Autodesk Inventor part; units mm, degrees
ref_plane "YZ Plane" through (0, 0, 0) normal (1, 0, 0) x (0, 1, 0)
ref_plane "XZ Plane" through (0, 0, 0) normal (0, 1, 0) x (-1, 0, 0)
ref_plane "XY Plane" through (0, 0, 0) normal (0, 0, 1) x (1, 0, 0)
sketch "Sketch1" plane through (0, 0, 0) normal (0, 0, 1) x (1, 0, 0)
  line L0 (0, 0) -> (25.6, 0)
  line L1 (25.6, 0) -> (25.6, -22)
  line L2 (25.6, -22) -> (0, -22)
  line L3 (0, -22) -> (0, 0)
  circle A0 centre (2.45, -19.55) radius 1.5
  line L4 (12.8, -22) -> (12.8, -20.4874)
  circle A1 centre (23.15, -19.55) radius 1.5
  circle A2 centre (5, -3.2) radius 1.5
  dimension "d0" = 25.6
  dimension "d1" = 22
  dimension "d2" = 3
  dimension "d3" = 2.45
  dimension "d4" = 2.45
  dimension "d5" = 3.2
  dimension "d6" = 3
extrude "Extrusion1" add sketch "Sketch1" along normal blind 2
properties part number "Plate_SEN_Current_sensor"
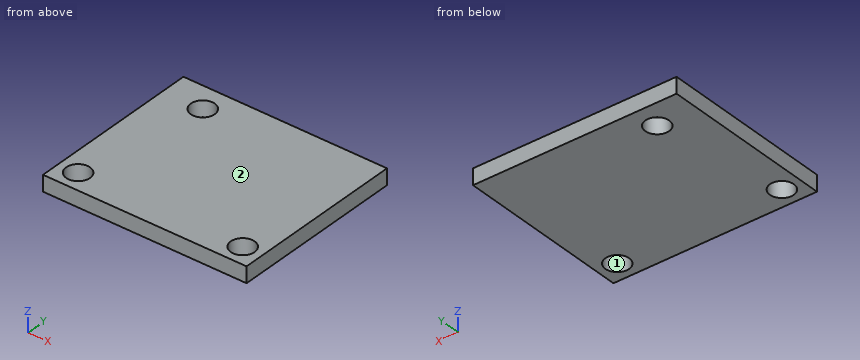
The model under review builds one solid part; all positions refer to its coordinate system, in mm. Face numbers are marked on the shaded views. Give positions to 0.01 mm unless a question says otherwise; leave off trailing zeros. Loops run counter-clockwise (first coordinate to the right, second up) from the corner with the lowest first, then second, coordinate; pieces in that order, holes last. Notation, with made-up numbers: (75.25, 86.25) -> (114.25, 86.25) arc R18 cw to (114.25, 103.25) -> close; hole circle Ø3 at (18, -18.75). An arc over 180 degrees is marked (long way). Use CSV: the item, a comma, the result in double quotes.
1. Consider section A-A, the plane y = -3.2. Write out the cut boundary in (x, z).
Result:
outline,"(0, 0) -> (3.5, 0) -> (3.5, 2) -> (0, 2) -> close; (6.5, 0) -> (25.6, 0) -> (25.6, 2) -> (6.5, 2) -> close"
2. To check wall thickness, follow probe 1 along Y at (x, z) = (23.15, 1); probe 2 along Y at (x, z) = (5, 1.55). State the ranges of each line that lie inside material, in increasing order. Write a range as from..to.
Result:
probe 1,"y = -22..-21.05, -18.05..0"
probe 2,"y = -22..-4.7, -1.7..0"
3. Consider section C-C, the plane y = -19.55. Write out the cut boundary in (x, z).
Result:
outline,"(0, 0) -> (0.95, 0) -> (0.95, 2) -> (0, 2) -> close; (3.95, 0) -> (21.65, 0) -> (21.65, 2) -> (3.95, 2) -> close; (24.65, 0) -> (25.6, 0) -> (25.6, 2) -> (24.65, 2) -> close"
4. The part is to be moulded in two halves that separate along Y. For the marked faces 1 and 2, say which applies: +Y half, -Y half, draft (parallel to the pull), parting line (faces both ways), or undercut.
Result:
face 1,"undercut"
face 2,"draft"
5. Consider section D-D, the plane z = 0.5. Write out the cut boundary in (x, y), then the cut area to 3 significant figures.
Result:
outline,"(0, -22) -> (25.6, -22) -> (25.6, 0) -> (0, 0) -> close; hole circle Ø3 at (2.45, -19.55); hole circle Ø3 at (5, -3.2); hole circle Ø3 at (23.15, -19.55)"
area,"542 mm²"
6. Consider section B-B, the plane x = 5. Write out the cut boundary in (y, z), then the cut area to 3 significant figures.
Result:
outline,"(-22, 0) -> (-4.7, 0) -> (-4.7, 2) -> (-22, 2) -> close; (-1.7, 0) -> (0, 0) -> (0, 2) -> (-1.7, 2) -> close"
area,"38.0 mm²"
7. For P1, Ø12, axis at x = 14.5, y = -19, coming from the -Z side, flat-tipped, find the tip position at first contact; note if it passes through.
Result:
P1,"stops at z = 0"
